Model file for the job. Use its own axes, mm. A direction names the side the tool comes from. Give positions to 0.01 mm unless a question says otherwise; leave off trailing zeros. Loops run counter-clockwise (first coordinate to the right, second up) from the corner with the lowest first, then second, coordinate; pieces in that order, holes last. Notation, with made-up numbers: (87, 79.25) -> (125, 79.25) arc R22 ccw to (125, 111.25) -> close; hole circle Ø11 at (10, 70). An arc over 180 degrees is marked (long way). Use CSV: the item, a comma, the result in double quotes. Start each with the question number.
(1) Cut at A-A on x = -316. Write the cut outline in (y, z).
(2) Pull direction X, two halves, no side cores. Call faces 1 (the flat face through (310, 1, 0)), 2 (the flat face through (-463, 1, 0)), 3 (the flat face through (-434.552, 57.257, 0.336)): pulls with the +X half, pulls with the -X half, needs draft (parallel to the pull), parting line crosses it, or undercut.
(3) Drill centre lines: probe 1 along X at (y, z) = (14.5, -18.5); probe 2 along X at (y, z) = (77.5, 4); probe 3 along X at (y, z) = (55, 10). Where is each one in solid material? Low to high.
(4) Cut at D-D on x = 60.5. Write the cut outline in (y, z).
(5) 3-axis set-ups, long thin cutter, end or side, ignore diameter. For faces 4 (the flat face through (-390, 48.2, 0)), 5 (the flat face through (-257, 9, 0)), 6 (the flat face through (-419.495, 21, 0)): which of +Z, -Z, +X, -X, +Y, -Y reach the whole face in a straight line?
(6) Flat gauge pins, fed straight in: pin 1 (14.5 mm diameter, centred on x = 451, z = 10, fed in from +Y); pin 2 (6 mm diameter, centred on y = 71.5, z = 0, fed in from -X); pin 3 (13 mm diameter, centred on y = 10.5, z = -9, fed in from +X); pin 4 (10 mm diameter, centred on x = 30, y = 32.5, fed in from +Z). Where does each tip first touch, or does it go through?
(7) Cut at B-B on z = -15. State how many separate pieces and enclosed holes the cut face has, then the cut area to 3 significant figures.
(8) Cut at C-C on y = 58. Write the cut outline in (x, z).
from build123d import *

# Parameters (mm, degrees)
SKETCH2_W           = 1010
SKETCH2_H           = 48
BOSS_EXTRUDE1_DEPTH = 1
SKETCH3_W           = 514
SKETCH3_H           = 48
BOSS_EXTRUDE2_DEPTH = 16
SKETCH4_W           = 56
SKETCH4_H           = 48
BOSS_EXTRUDE3_DEPTH = 41.2
EXTRUDE_THIN1_DEPTH = 48


with BuildPart() as part:
    # Sketch2 → Boss-Extrude1 (new body)
    with BuildSketch(Plane(origin=(0, 0, 0), x_dir=(1, 0, 0), z_dir=(0, 1, 0))):
        Rectangle(SKETCH2_W, SKETCH2_H)
    extrude(amount=BOSS_EXTRUDE1_DEPTH)

    # Sketch3 → Boss-Extrude2 (add)
    with BuildSketch(Plane(origin=(0, 1, 0), x_dir=(1, 0, 0), z_dir=(0, 1, 0))):
        Rectangle(SKETCH3_W, SKETCH3_H)
    extrude(amount=BOSS_EXTRUDE2_DEPTH)

    # Sketch4 → Boss-Extrude3 (add)
    with BuildSketch(Plane(origin=(0, 1, 0), x_dir=(1, 0, 0), z_dir=(0, 1, 0))):
        with Locations((-391.494906848, 0)):
            Rectangle(SKETCH4_W, SKETCH4_H)
    boss_extrude3 = extrude(amount=BOSS_EXTRUDE3_DEPTH)

    # Mirror1: Boss-Extrude3 across plane
    add(boss_extrude3.mirror(Plane(origin=(0, 0, 0), x_dir=(0, 0, 1), z_dir=(1, 0, 0))))

    # Sketch7 → Extrude-Thin1 (add)
    with BuildSketch(Plane.XY.offset(24)):
        Polygon((-431.515722128, 89.576154339), (-449.193391658, 71.89848481), (-419.494906848, 42.2), (-363.494906848, 42.2), (-257, 17), (257, 17), (363.494906848, 42.2), (419.494906848, 42.2), (449.193391658, 71.89848481), (431.515722128, 89.576154339), (427.273081441, 85.333513652), (440.708110284, 71.89848481), (417.009625474, 48.2), (362.794682376, 48.2), (256.299775528, 23), (-256.299775528, 23), (-362.794682376, 48.2), (-417.009625474, 48.2), (-440.708110284, 71.89848481), (-427.273081441, 85.333513652), align=None)
    extrude(amount=-EXTRUDE_THIN1_DEPTH)


solid = part.part
Check result:
1,outline,"(0, -24) -> (1, -24) -> (1, 24) -> (0, 24) -> close; (30.96, -24) -> (37.13, -24) -> (37.13, 24) -> (30.96, 24) -> close"
2,face 1,"undercut"
2,face 2,"needs draft"
2,face 3,"pulls with the -X half"
3,probe 1,"-419.49 to -363.49, -257 to 257, 363.49 to 419.49"
3,probe 2,"-443.59 to -435.11, 435.11 to 443.59"
3,probe 3,"-432.29 to -423.81, 423.81 to 432.29"
4,outline,"(0, -24) -> (23, -24) -> (23, 24) -> (0, 24) -> close"
5,face 4,"+Z, -Z, +Y"
5,face 5,"+Z, -Z"
5,face 6,"+Z, -Z, -X"
6,pin 1,"y = 77.34"
6,pin 2,"x = -449.19"
6,pin 3,"x = 419.49"
6,pin 4,"through"
7,separate pieces,"1"
7,enclosed holes,"2"
7,area,"19,600 mm²"
8,outline,"(-435.29, -24) -> (-426.81, -24) -> (-426.81, 24) -> (-435.29, 24) -> close; (426.81, -24) -> (435.29, -24) -> (435.29, 24) -> (426.81, 24) -> close"
